Source: three-view drawing plus pictorial views. Frame: mm from the lowest corner of the part. Give positions to 0.01 mm unless a question says otherwise; leave off trailing zeros. Write each loop counter-clockwise with the first axis right and the second up, starting at its lowest first coordinate (ties: lowest second). Pieces come first, ordered by that corner, then holes.
Q1. Cut plane B-B on x = 23. Return the cut outline in (y, z).
Q2. Pin query (flat end, axial travel): pin 1 (4.5 mm diameter, centred on x = 5, y = 13, fed in from -Z). Return the tip coordinate at first contact, or that it passes through.
Q3. Cut plane D-D on z = 0.65. Return the cut outline in (x, y).
Q4. Cut plane A-A on y = 23. Return the cut outline in (x, z).
Q5. Draft query along Y for the marked faces 1, 2 and 3. Return one class per face: pulls with the +Y half, pulls with the -Y half, needs draft (parallel to the pull), parting line crosses it, or undercut.
Q6. Line query: L1, parallel to Y at x = 19, z = 2.1; L2, parallel to Y at x = 3.75, z = 0.75; L3, parallel to Y at x = 23, z = 0.8. Output: solid intervals per line, ascending.
Q7. Cut plane C-C on x = 5. Return the cut outline in (y, z), plus the area to 3 significant figures.
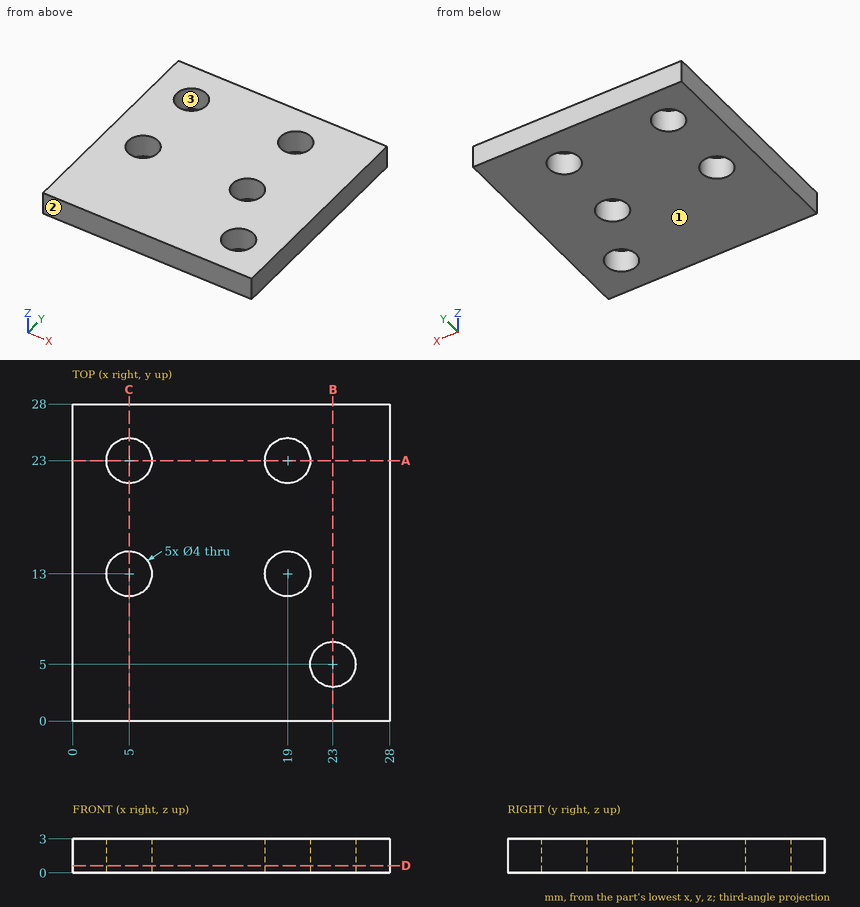
Data:
1. outline: (0, 0) - (3, 0) - (3, 3) - (0, 3) - close; (7, 0) - (28, 0) - (28, 3) - (7, 3) - close
2. pin 1: stops at z = 0
3. outline: (0, 0) - (28, 0) - (28, 28) - (0, 28) - close; hole circle Ø4 at (5, 13); hole circle Ø4 at (5, 23); hole circle Ø4 at (19, 13); hole circle Ø4 at (19, 23); hole circle Ø4 at (23, 5)
4. outline: (0, 0) - (3, 0) - (3, 3) - (0, 3) - close; (7, 0) - (17, 0) - (17, 3) - (7, 3) - close; (21, 0) - (28, 0) - (28, 3) - (21, 3) - close
5. face 1: needs draft
5. face 2: pulls with the -Y half
5. face 3: undercut
6. L1: y = 0 to 11, 15 to 21, 25 to 28
6. L2: y = 0 to 11.44, 14.56 to 21.44, 24.56 to 28
6. L3: y = 0 to 3, 7 to 28
7. outline: (0, 0) - (11, 0) - (11, 3) - (0, 3) - close; (15, 0) - (21, 0) - (21, 3) - (15, 3) - close; (25, 0) - (28, 0) - (28, 3) - (25, 3) - close
7. area: 60.0 mm2
